Input: part model. Units: mm. Frame: model coordinates. Face numbers are marked on the shaded views. A direction names the side the tool comes from. Coordinates: 2 decimals unless noted, no trailing zeros. Order: outer loops, then holes, each group sorted by start corner. A loop starts at its lowest first (then second) coordinate and runs counter-clockwise, first axis right, second up. Notation, with made-up numbers: M -4,60 L 17,60 A15 cw 17,89 Z; hole C 43,7.25 d7. An arc over 180 degrees is marked long. Answer in a Markdown table with one row per item.
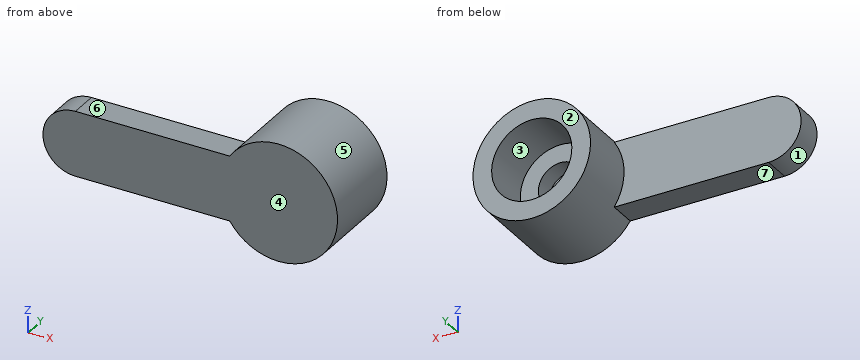
from build123d import *

# Parameters (mm, degrees)
SKETCH1_R           = 2.125
BOSS_EXTRUDE1_DEPTH = 3.1
SKETCH2_R           = 1.45
CUT_EXTRUDE1_DEPTH  = 1.8
SKETCH3_R           = 0.8
CUT_EXTRUDE2_DEPTH  = 0.65
BOSS_EXTRUDE3_DEPTH = 1


with BuildPart() as part:
    # Sketch1 → Boss-Extrude1 (new body)
    with BuildSketch(Plane(origin=(0, 0, 0), x_dir=(1, 0, 0), z_dir=(0, 1, 0))):
        with Locations(Location((0, 0, 0), (0, 0, 90))):
            Circle(SKETCH1_R)
    extrude(amount=BOSS_EXTRUDE1_DEPTH)

    # Sketch2 → Cut-Extrude1 (cut)
    with BuildSketch(Plane(origin=(0, 3.1, 0), x_dir=(1, 0, 0), z_dir=(0, 1, 0))):
        with Locations(Location((0, 0, 0), (0, 0, 270))):
            Circle(SKETCH2_R)
    extrude(amount=-CUT_EXTRUDE1_DEPTH, mode=Mode.SUBTRACT)

    # Sketch3 → Cut-Extrude2 (cut)
    with BuildSketch(Plane(origin=(0, 1.3, 0), x_dir=(1, 0, 0), z_dir=(0, 1, 0))):
        with Locations(Location((0, 0, 0), (0, 0, 270))):
            Circle(SKETCH3_R)
    extrude(amount=-CUT_EXTRUDE2_DEPTH, mode=Mode.SUBTRACT)

    # Sketch4 → Boss-Extrude3 (add)
    with BuildSketch(Plane(origin=(0, 0, 0), x_dir=(1, 0, 0), z_dir=(0, 1, 0))):
        with BuildLine():
            Line((-1.770593121, -1.175), (-7.35, -1.175))
            ThreePointArc((-7.35, -1.175), (-8.525, 0), (-7.35, 1.175))
            Line((-7.35, 1.175), (-1.770593121, 1.175))
            ThreePointArc((-1.770593121, 1.175), (-2.125, 0), (-1.770593121, -1.175))
        make_face()
    extrude(amount=BOSS_EXTRUDE3_DEPTH)


solid = part.part
1) Cut plane D-D, the plane y = 1.55. Output: boundary loops of the cut face in (x, z) (3 decimals).
Resolved:
| item | result |
|---|---|
| outline | C 0,0 d4.25; hole C 0,0 d2.9 |
2) Cut plane A-A, the plane y = 0.85. Output: boundary loops of the cut face in (x, z) (3 decimals).
Resolved:
| item | result |
|---|---|
| outline | M -7.35,-1.175 L -1.771,-1.175 A2.125 ccw long -1.771,1.175 L -7.35,1.175 A1.175 ccw Z; hole C 0,0 d1.6 |
3) Cut plane B-B, the plane x = 0. Output: boundary loops of the cut face in (y, z) (3 decimals).
Resolved:
| item | result |
|---|---|
| outline | M 0,-2.125 L 3.1,-2.125 L 3.1,-1.45 L 1.3,-1.45 L 1.3,-0.8 L 0.65,-0.8 L 0.65,0.8 L 1.3,0.8 L 1.3,1.45 L 3.1,1.45 L 3.1,2.125 L 0,2.125 Z |
4) Cut plane C-C, the plane z = 0. Output: boundary loops of the cut face in (x, y) (3 decimals).
Resolved:
| item | result |
|---|---|
| outline | M -8.525,0 L 2.125,0 L 2.125,3.1 L 1.45,3.1 L 1.45,1.3 L 0.8,1.3 L 0.8,0.65 L -0.8,0.65 L -0.8,1.3 L -1.45,1.3 L -1.45,3.1 L -2.125,3.1 L -2.125,1 L -8.525,1 Z |
5) Material intervals for probe 1 along X at (y, z) = (2, -0.65); probe 2 along Z at (x, y) = (-0.5, 1.6); probe 3 along X at (y, z) = (1.8, 0) (3 decimals), sorted ascending.
Resolved:
| item | result |
|---|---|
| probe 1 | x = -2.02 to -1.3, 1.3 to 2.02 |
| probe 2 | z = -2.07 to -1.36, 1.36 to 2.07 |
| probe 3 | x = -2.125 to -1.45, 1.45 to 2.125 |
6) Reachability of the marked faces 4, 5, 6 and 7 from +Z, -Z, +X, -X, +Y, -Y: full face, straight path, thin tool, end or side. Return the list, or none.
Resolved:
| item | result |
|---|---|
| face 4 | +Z, -Z, +X, -X, -Y |
| face 5 | +Y |
| face 6 | +Z, -X, +Y, -Y |
| face 7 | -Z, -X, +Y, -Y |
7) Mould query, pull axis X, two halves, no side actions, for the marked faces 1, 2 and 3. Classes: +X half, -X half, draft (parallel to the pull), parting line (faces both ways), or undercut.
Resolved:
| item | result |
|---|---|
| face 1 | -X half |
| face 2 | draft |
| face 3 | undercut |
8) Contact query for flat-ended pins moving along their axis: pin 1 (1 mm diameter, centred on y = 1.5, z = 1.5, fed in from +X) (3 decimals); pin 2 (0.5 mm diameter, centred on x = -3.5, y = 0.5, fed in from +Z) (3 decimals); pin 3 (1.5 mm diameter, centred on x = -0.5, z = 1, fed in from +Y); pin 4 (1 mm diameter, centred on x = -7.5, z = 1.5, fed in from +Y). Output: stop coordinate, or through.
Resolved:
| item | result |
|---|---|
| pin 1 | stops at x = 1.875 |
| pin 2 | stops at z = 1.175 |
| pin 3 | stops at y = 3.1 |
| pin 4 | stops at y = 1 |
